For this review, take the finished solid that the model builds, in its own axes (mm). A direction names the side the tool comes from. Coordinates: 2 decimals unless noted, no trailing zeros. Write each loop counter-clockwise with the first axis right and the second up, starting at its lowest first coordinate (ties: lowest second). Pieces come first, ordered by that corner, then holes. Notation, with made-up numbers: M -27.5,67 L -18.5,67 A11 ccw -18.5,85 Z; hole C 65,24.5 d3. An arc over 180 degrees is marked long. Return JSON: item names as keys, results as strings.
```python
from build123d import *

# Parameters (mm, degrees)
SKETCH1_R           = 165.1
SKETCH1_R_2         = 88.9
BOSS_EXTRUDE1_DEPTH = 152.4
FILLET1_R           = 12.7
SHELL2_START        = 12.7
SHELL2_OUTLINE_R    = 152.4
SHELL2_OUTLINE_R_2  = 101.6
SHELL2_DEPTH        = 127


# Read off the part's stored shape, not the designer's step: Shell2
with BuildPart() as part:
    # Sketch1 → Boss-Extrude1 (new body)
    with BuildSketch(Plane(origin=(0, 0, 0), x_dir=(0, 0, -1), z_dir=(1, 0, 0))):
        with Locations(Location((0, 0, 0), (0, 0, 180))):
            Circle(SKETCH1_R)
        with Locations(Location((0, 0, 0), (0, 0, 180))):
            Circle(SKETCH1_R_2, mode=Mode.SUBTRACT)
    extrude(amount=BOSS_EXTRUDE1_DEPTH)

    # Fillet1
    fillet1_edges = [part.edges().sort_by_distance(p)[0] for p in [
        (0, 0, -165.1),
        (152.4, 0, -165.1),
    ]]
    fillet(fillet1_edges, radius=FILLET1_R)

    # Shell2 outline → Shell2 (cut)
    with BuildSketch(Plane.YZ.offset(SHELL2_START)):
        Circle(SHELL2_OUTLINE_R)
        Circle(SHELL2_OUTLINE_R_2, mode=Mode.SUBTRACT)
    extrude(amount=SHELL2_DEPTH, mode=Mode.SUBTRACT)


solid = part.part
```
1. Wall thickness on L1, parallel to X at y = -24, z = 103; L2, parallel to Z at x = 69, y = -90; L3, parallel to Y at x = 86, z = -11: over which ranges is each line inside the solid? List them lowest first. Write a range as from..to.
Checks:
{"L1": "0..12.7, 139.7..152.4", "L2": "-138.41..-122.99, -47.14..47.14, 122.99..138.41", "L3": "-164.73..-152, -101..-88.22, 88.22..101, 152..164.73"}
2. For faces 4 (the face through (139.7, 32, -99)), 5 (the face through (0, 66, 66)), list the 3-axis set-ups (+Z, -Z, +X, -X, +Y, -Y) from which the entire face can be reached by the end or side of a thin tool; tool diameter is ignored.
Checks:
{"face 4": "none", "face 5": "+Z, -Z, -X, +Y, -Y"}
3. We need section A-A (y = 0). State the section outline as (x, z) points.
Checks:
{"outline": "M 0,-152.4 A12.7 ccw 12.7,-165.1 L 139.7,-165.1 A12.7 ccw 152.4,-152.4 L 152.4,-88.9 L 0,-88.9 Z; M 0,88.9 L 152.4,88.9 L 152.4,152.4 A12.7 ccw 139.7,165.1 L 12.7,165.1 A12.7 ccw 0,152.4 Z; hole M 12.7,-152.4 L 139.7,-152.4 L 139.7,-101.6 L 12.7,-101.6 Z; hole M 12.7,101.6 L 139.7,101.6 L 139.7,152.4 L 12.7,152.4 Z"}
4. We need section D-D (y = -96). Give the number of separate pieces and of enclosed holes in the cut face, plus the area to 3 significant figures.
Checks:
{"separate pieces": "1", "enclosed holes": "2", "area": "19,200 mm2"}
5. We need section C-C (x = 21). State the section outline as (y, z) points, plus the area to 3 significant figures.
Checks:
{"outline": "C 0,0 d330.2; C 0,0 d203.2; hole C 0,0 d304.8; hole C 0,0 d177.8", "area": "20,300 mm2"}
6. Draft analysis for pull direction Z (two halves, no side actions). For faces 1 (the face through (152.4, 66, 66)), 2 (the face through (75.133, -60.083, -65.523)), 3 (the face through (75.311, -163.695, -21.493)), state which applies: +Z half, -Z half, draft (parallel to the pull), parting line (faces both ways), or undercut.
Checks:
{"face 1": "draft", "face 2": "undercut", "face 3": "parting line"}
7. Clearance check with flat-ended pins moving along their axes: pin 1 Ø1.5 at (y, z) = (-124, -20) entering from -X; pin 2 Ø6 at (x, z) = (62, -18) entering from -Y; pin 3 Ø2 at (x, y) = (99.5, -88.5) entering from +Z; pin 4 Ø1.5 at (x, y) = (66.5, 98) entering from +Z. State where each tip first meets the part, or that it passes through.
Checks:
{"pin 1": "x = 0", "pin 2": "y = -164.42", "pin 3": "z = 140.01", "pin 4": "z = 133.42"}
